Verification items for the finished model (mm, model axes). A direction names the side the tool comes from. Coordinates: 2 decimals unless noted, no trailing zeros. Loops run counter-clockwise (first coordinate to the right, second up) from the corner with the lowest first, then second, coordinate; pieces in that order, holes last.
Q1. Go/stop test with flat-tipped pins: P1, Ø3, axis at x = 4.5, z = 7, coming from the -Y side; P2, Ø2, axis at x = -1.5, z = 2.5, coming from the +Y side; P3, Ø3, axis at x = -12.5, y = 0, coming from the -Z side; P4, Ø2, axis at x = -0.5, z = 3.5, coming from the -Y side. Record where each tip stops, or that it passes through.
Q2. Sectioned sample at C-C (y = 0). Enter the section's corners in (x, z).
Q3. Sectioned sample at B-B (z = 3.5). Enter the section's corners in (x, y).
Q4. Mould release check, pull along X, two halves, no side actions. Record for faces 4 (the face through (7.27, 3.09, 5.47)), 5 (the face through (-7.68, -0.26, -2.1)), 6 (the face through (0.776, -1.879, 7.071)): +X half, -X half, draft (parallel to the pull), parting line (faces both ways), or undercut.
Q5. Sectioned sample at A-A (x = -12.5). Enter the section's corners in (y, z).
Q6. Sectioned sample at D-D (x = -8.5). Enter the section's corners in (y, z), then the cut area to 4 significant figures.
Q7. Material ranges on probe 1 along Y at (x, z) = (12.5, 0.6); probe 2 along X at (y, z) = (-0.5, 0.5); probe 3 along Z at (x, y) = (0, 0), recorded low to high.
Q8. Access from +Z, -Z, +X, -X, +Y, -Y to the whole of each face (thin tool, end or side, straight path). Record for faces 1 (the face through (14.97, 5.8, 0.46)), 2 (the face through (-0.098, 2.166, 7.071)), 3 (the face through (7.67, -0.33, 2.91)).
```python
from build123d import *

# Parameters (mm, degrees)
F0_W      = 30.8
F0_H      = 12.5
F1_DEPTH  = 0.9
F2_R      = 1.5
F4_DEPTH  = 5.16
F5_R      = 1.7
F6_SIZE   = 1.2
F7_R      = 0.75
F8_DEPTH  = 2.05
F9_R      = 1.55
F10_DEPTH = 0.9


with BuildPart() as f1:
    # F0 (on Top) → F1 (new body)
    with BuildSketch(Plane.XY):
        Rectangle(F0_W, F0_H)
    extrude(amount=F1_DEPTH)

    # F2
    f2_edges = [f1.edges().sort_by_distance(p)[0] for p in [
        (-15.4, 6.25, 0.45),
        (15.4, 6.25, 0.45),
        (15.4, -6.25, 0.45),
        (-15.4, -6.25, 0.45),
    ]]
    fillet(f2_edges, radius=F2_R)

    # F3 (on face) → F4 (join, symmetric)
    with BuildSketch(Plane.XY.offset(0.9)):
        Polygon((8.45, 4.1), (-8.45, 4.1), (-7.0041187582, -4.1), (7.0041187582, -4.1), align=None)
    extrude(amount=F4_DEPTH, both=True)

    # F5
    f5_edges = [f1.edges().sort_by_distance(p)[0] for p in [
        (-8.45, 4.1, -2.13),
        (-8.45, 4.1, 3.48),
        (8.45, 4.1, -2.13),
        (8.45, 4.1, 3.48),
        (-7.004119, -4.1, -2.13),
        (-7.004119, -4.1, 3.48),
        (7.004119, -4.1, -2.13),
        (7.004119, -4.1, 3.48),
    ]]
    fillet(f5_edges, radius=F5_R)

    # F6
    f6_edges = [f1.edges().sort_by_distance(p)[0] for p in [
        (0, 4.1, 6.06),
    ]]
    chamfer(f6_edges, length=F6_SIZE)

    # F7 (on face) → F8 (join)
    with BuildSketch(Plane.XY.offset(6.06)):
        with Locations((-5.4864, 1.4224)):
            Circle(F7_R)
        with Locations((-2.7432, 1.4224)):
            Circle(F7_R)
        with Locations((0, 1.4224)):
            Circle(F7_R)
        with Locations((2.7432, 1.4224)):
            Circle(F7_R)
        with Locations((5.4864, 1.4224)):
            Circle(F7_R)
        with Locations((4.1148, -1.4224)):
            Circle(F7_R)
        with Locations((1.3716, -1.4224)):
            Circle(F7_R)
        with Locations((-1.3716, -1.4224)):
            Circle(F7_R)
        with Locations((-4.1148, -1.4224)):
            Circle(F7_R)
    extrude(amount=F8_DEPTH)

    # F9 (on face) → F10 (cut)
    with BuildSketch(Plane.XY.offset(0.9)):
        with Locations((-12.5, 0)):
            Circle(F9_R)
        with Locations((12.5, 0)):
            Circle(F9_R)
    extrude(amount=-F10_DEPTH, mode=Mode.SUBTRACT)


solid = f1.part
```
Geometry check:
1. P1: stops at y = -3.46
1. P2: stops at y = 4.1
1. P3: passes through
1. P4: stops at y = -4.1
2. outline: (-15.4, 0) - (-14.05, 0) - (-14.05, 0.9) - (-15.4, 0.9) - close; (-10.95, 0) - (-7.73, 0) - (-7.73, -4.26) - (7.73, -4.26) - (7.73, 0) - (10.95, 0) - (10.95, 0.9) - (7.73, 0.9) - (7.73, 4.86) - (6.51, 6.06) - (-6.51, 6.06) - (-7.73, 4.86) - (-7.73, 0.9) - (-10.95, 0.9) - close; (14.05, 0) - (15.4, 0) - (15.4, 0.9) - (14.05, 0.9) - close
3. outline: (-8.1, 2.1) - (-7.25, -2.7) arc R1.7 ccw to (-5.58, -4.1) - (5.58, -4.1) arc R1.7 ccw to (7.25, -2.7) - (8.1, 2.1) arc R1.7 ccw to (6.42, 4.1) - (-6.42, 4.1) arc R1.7 ccw to start
4. face 4: +X half
4. face 5: -X half
4. face 6: undercut
5. outline: (-6.25, 0) - (-1.55, 0) - (-1.55, 0.9) - (-6.25, 0.9) - close; (1.55, 0) - (6.25, 0) - (6.25, 0.9) - (1.55, 0.9) - close
6. outline: (-6.25, 0) - (6.25, 0) - (6.25, 0.9) - (-6.25, 0.9) - close
6. area: 11.25 mm2
7. probe 1: y = -6.25 to -1.55, 1.55 to 6.25
7. probe 2: x = -15.4 to -13.97, -11.03 to 11.03, 13.97 to 15.4
7. probe 3: z = -4.26 to 6.06
8. face 1: +Z, -Z, +X, +Y
8. face 2: +Z
8. face 3: +Z, +X, -Y
